Here's the drawing with two shaded views (mm, measured from the low corner). I have some questions. Round coordinates to 2 decimals unless told otherwise and drop trailing zeros. Loops run counter-clockwise (first coordinate to the right, second up) from the corner with the lowest first, then second, coordinate; pieces in that order, holes last. Notation, with made-up numbers: M 17.5,27 L 28.5,27 A21 cw 28.5,42 Z; hole C -1.5,61.5 d9. An arc over 180 degrees is marked long. One line per item, written item: value. Start each with the question number.
Q1. Imagine slicing it at D-D (x = 56). Please give me the cut outline in (y, z).
Q2. Please list where these lines run through material, in increasing order: line 1 along X through (y, z) = (22.5, 25); line 2 along X through (y, z) = (6, 22.5); line 3 along Y through (x, z) = (63.5, 42.5).
Q3. Imagine slicing it at B-B (x = 30). Please give me the cut outline in (y, z).
Q4. Thinking about a two-plate mould opening in X: for the marked faces 1 and 2, which applies, released by +X, released by -X, zero draft, split by the parting line, or undercut?
Q5. Imagine slicing it at C-C (y = 7). Please give me the cut outline in (x, z).
Q6. I'm going to push flat-ended pins straight in: pin 1 Ø3 at (x, z) = (120, 25) entering from +Y; pin 2 Ø8.5 at (x, z) = (120, 25) entering from -Y; pin 3 Ø5 at (x, z) = (30, 25) entering from -Y; pin 4 Ø10 at (y, z) = (2.5, 28) entering from +X. Where does each tip first touch, or does it pass through?
Q7. Imagine slicing it at A-A (z = 25). Give the number of separate pieces and of enclosed holes in the cut face, then the cut area to 3 significant figures.
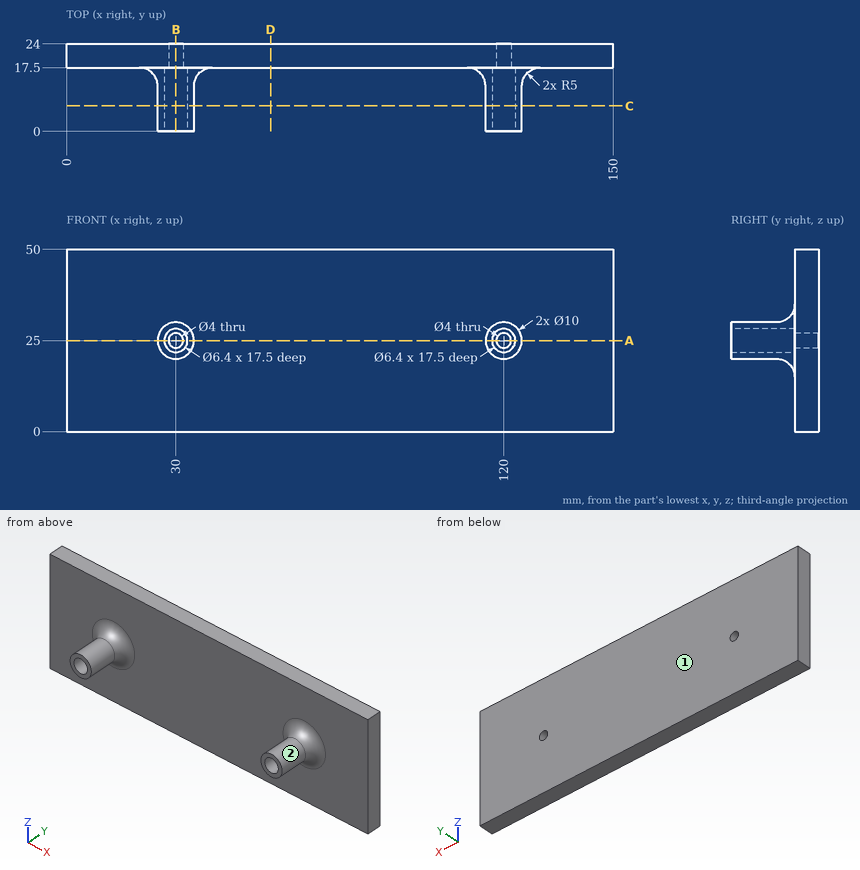
Report:
1. outline: M 17.5,0 L 24,0 L 24,50 L 17.5,50 Z
2. line 1: x = 0 to 28, 32 to 118, 122 to 150
2. line 2: x = 25.67 to 28, 32 to 34.33, 115.67 to 118, 122 to 124.33
2. line 3: y = 17.5 to 24
3. outline: M 0,20 L 12.5,20 A5 cw 17.5,15 L 17.5,0 L 24,0 L 24,23 L 17.5,23 L 17.5,21.8 L 0,21.8 Z; M 0,28.2 L 17.5,28.2 L 17.5,27 L 24,27 L 24,50 L 17.5,50 L 17.5,35 A5 cw 12.5,30 L 0,30 Z
4. face 1: zero draft
4. face 2: undercut
5. outline: C 30,25 d10; C 120,25 d10; hole C 30,25 d6.4; hole C 120,25 d6.4
6. pin 1: passes through
6. pin 2: stops at y = 0
6. pin 3: stops at y = 17.5
6. pin 4: stops at x = 125
7. separate pieces: 3
7. enclosed holes: 0
7. area: 1,070 mm²
